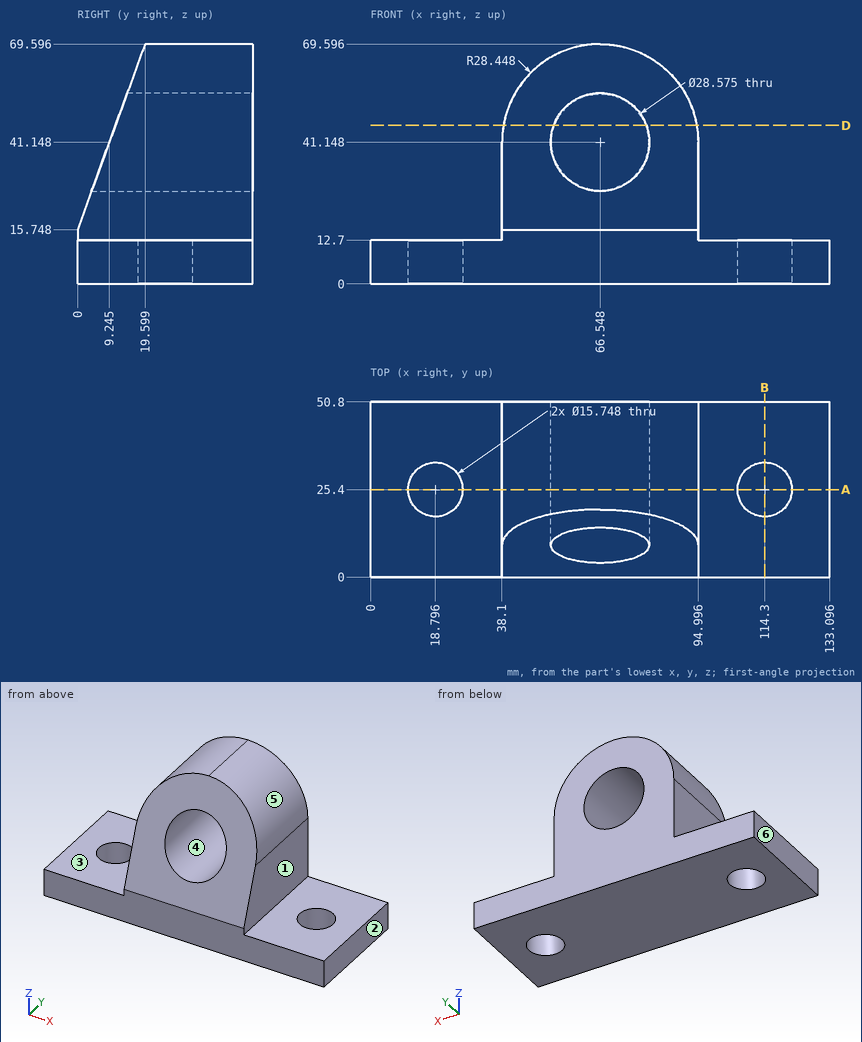
Here's the drawing with two shaded views (mm, measured from the low corner). I have some questions. A direction names the side the tool comes from. Coordinates: 2 decimals unless noted, no trailing zeros. Order: outer loops, then holes, each group sorted by start corner. A loop starts at its lowest first (then second) coordinate and runs counter-clockwise, first axis right, second up. Notation, with made-up numbers: M -27.75,23.25 L 28.25,23.25 A16 ccw 28.25,53.25 Z; hole C 64,7 d11. An arc over 180 degrees is marked long. Answer as CSV lines item,"result".
Item 1: Imagine slicing it at D-D on z = 46. Write out the boundary of the cut face in (x, y).
Results found:
outline,"M 38.52,11.01 L 53.11,11.01 L 53.11,50.8 L 38.52,50.8 Z; M 79.99,11.01 L 94.58,11.01 L 94.58,50.8 L 79.99,50.8 Z"
Item 2: Imagine slicing it at A-A on y = 25.4. Give the number of separate pieces and of enclosed holes in the cut face, plus the area to 3 significant figures.
Results found:
separate pieces,"3"
enclosed holes,"1"
area,"3,540 mm2"
Item 3: On a 3-axis mill with a long thin cutter (end or side, diameter ignored), from which of +Z, -Z, +X, -X, +Y, -Y can I reach the whole of each face in a straight line? I mean the marked faces 1, 2 and 3. Say none if no direction works.
Results found:
face 1,"+Z, +X, +Y, -Y"
face 2,"+Z, -Z, +X, +Y, -Y"
face 3,"+Z, -X, +Y, -Y"
Item 4: We'd pull the mould along Z, two halves only. Please class the marked faces 4, 5 and 6: +Z half, -Z half, draft (parallel to the pull), parting line (faces both ways), or undercut.
Results found:
face 4,"undercut"
face 5,"+Z half"
face 6,"draft"
Item 5: Imagine slicing it at B-B on x = 114.3. Write out the boundary of the cut face in (y, z).
Results found:
outline,"M 0,0 L 17.53,0 L 17.53,12.7 L 0,12.7 Z; M 33.27,0 L 50.8,0 L 50.8,12.7 L 33.27,12.7 Z"
Item 6: If I drill on line 1 (X direction, y = 25, z = 7); line 2 (X direction, y = 32, z = 9) (1 decimal); line 3 (Z direction, x = 15, y = 48), over which ranges is the centre line in solid material (lowest first)?
Results found:
line 1,"0 to 10.93, 26.66 to 106.44, 122.16 to 133.1"
line 2,"0 to 14.5, 23.1 to 110, 118.6 to 133.1"
line 3,"0 to 12.7"
Item 7: For pin 1 (5 mm diameter, centred on x = 101.5, z = 14, fed in from +Y); pin 2 (10 mm diameter, centred on x = 105, y = 25.5, fed in from +Z); pin 3 (23 mm diameter, centred on y = 31, z = 27.5, fed in from +X), each with a flat end and sliding along its axis, tell me the tip position at first contact or that it passes through.
Results found:
pin 1,"y = 50.8"
pin 2,"z = 12.7"
pin 3,"x = 95"
